Model file for the job. Use its own axes, mm. Face numbers are marked on the shaded views. Coordinates: 2 decimals unless noted, no trailing zeros. Loops run counter-clockwise (first coordinate to the right, second up) from the corner with the lowest first, then second, coordinate; pieces in that order, holes last. Notation, with made-up numbers: (56.5, 76) -> (111.5, 76) arc R13 ccw to (111.5, 84) -> close; hole circle Ø7 at (-6.5, 80.25). An arc over 180 degrees is marked (long way). Use one line per item in the form item = value.
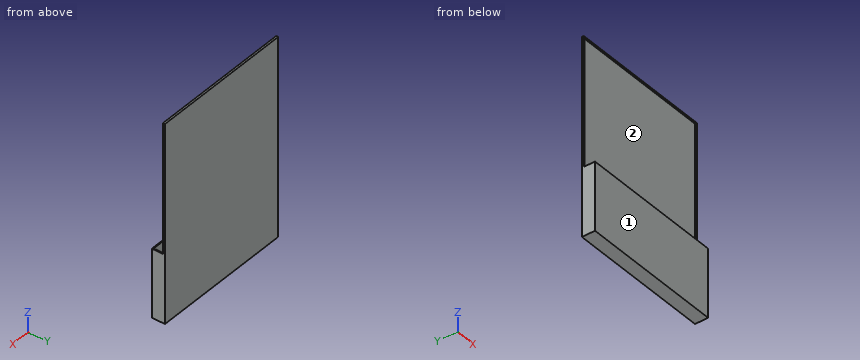
```python
from build123d import *

# Parameters (mm, degrees)
F0_W     = 220
F0_H     = 103.788202
F1_DEPTH = 20
F0_H_2   = 196.211798
F2_DEPTH = 3
F3_T     = -1.5


with BuildPart() as f1:
    # F0 (on Front) → F1 (new body)
    with BuildSketch(Plane.XZ):
        with Locations((0, -98.105899)):
            Rectangle(F0_W, F0_H)
    extrude(amount=F1_DEPTH)

    # F0 (on Front) → F2 (join)
    with BuildSketch(Plane.XZ):
        with Locations((0, 51.894101)):
            Rectangle(F0_W, F0_H_2)
    extrude(amount=F2_DEPTH)

    # F3
    f3_openings = [f1.faces().sort_by_distance(p)[0] for p in [
        (0, -11.5, -46.211798),
        (0, -3, 51.894101),
    ]]
    offset(amount=F3_T, openings=f3_openings)


solid = f1.part
```
Q1. Pin check, flat tips, straight feed: pin 1 Ø5 at (x, z) = (68, -10.5) entering from -Y; pin 2 Ø8.5 at (x, y) = (-21.5, -13) entering from +Z. Stop position of each tip, or through.
Result:
pin_1 = -1.5
pin_2 = -148.5
Q2. Band-saw the part on A-A, the plane x = 51. Write the cut outline in (y, z).
Result:
outline = (-20, -150) -> (0, -150) -> (0, 150) -> (-3, 150) -> (-3, 148.5) -> (-1.5, 148.5) -> (-1.5, -148.5) -> (-18.5, -148.5) -> (-18.5, -46.21) -> (-20, -46.21) -> close
Q3. Mould opens along Z. For the marked faces 1 and 2 say: released by +Z, released by -Z, zero draft, split by the parting line, or undercut.
Result:
face_1 = zero draft
face_2 = undercut
Q4. Wall check: line 1 along Y through (x, z) = (14, -125.5); line 2 along X through (y, z) = (-2, 29.5); line 3 along Z through (x, y) = (-85, -17.25). Give the ranges that are in metal, low to high.
Result:
line_1 = -20 to -18.5, -1.5 to 0
line_2 = -110 to -108.5, 108.5 to 110
line_3 = -150 to -148.5
Q5. Band-saw the part on C-C, the plane y = -12.5. Write the cut outline in (x, z).
Result:
outline = (-110, -150) -> (110, -150) -> (110, -46.21) -> (108.5, -46.21) -> (108.5, -148.5) -> (-108.5, -148.5) -> (-108.5, -46.21) -> (-110, -46.21) -> close
Q6. Band-saw the part on B-B, the plane z = -112.5. Write the cut outline in (x, y).
Result:
outline = (-110, -20) -> (110, -20) -> (110, 0) -> (-110, 0) -> close; hole (-108.5, -18.5) -> (108.5, -18.5) -> (108.5, -1.5) -> (-108.5, -1.5) -> close
Q7. Band-saw the part on D-D, the plane z = 60. Write the cut outline in (x, y), and give its area (4 significant figures).
Result:
outline = (-110, -3) -> (-108.5, -3) -> (-108.5, -1.5) -> (108.5, -1.5) -> (108.5, -3) -> (110, -3) -> (110, 0) -> (-110, 0) -> close
area = 334.5 mm2
